Source: CAD feature listing. Evaluate the final solid. Frame: model axes, mm. A direction names the side the tool comes from. Round coordinates to 2 decimals unless told otherwise and drop trailing zeros. Loops run counter-clockwise (first coordinate to the right, second up) from the corner with the lowest first, then second, coordinate; pieces in that order, holes last. Notation, with made-up numbers: (-24, -5.5) - (-1, -5.5) arc R12 ccw to (-1, 12.5) - close; hole circle Ø4 at (3.25, 27.5). An arc over 180 degrees is marked (long way). One line per question, with ' | ' between items. Start each with the question number.
1. Pin query (flat end, axial travel): pin 1 (4 mm diameter, centred on x = 20.5, z = 22, fed in from -Y); pin 2 (1 mm diameter, centred on x = 5, y = 5.5, fed in from +Z); pin 3 (4.5 mm diameter, centred on x = 16.5, y = -2, fed in from +Z); pin 4 (4.5 mm diameter, centred on x = 16.5, y = 0, fed in from -Z). Return the tip coordinate at first contact, or that it passes through.
2. Cut plane B-B (z = 8). Return loops of the section in (x, y).
3. Cut plane A-A (x = 23.5). Return loops of the section in (y, z), then the cut area to 3 significant figures.
4. Mould query, pull axis Y, two halves, no side actions, for faces 1 (the flat face through (15, -2, 27)), 2 (the cylindrical face through (21.32, -7.58, 7.94)), 3 (the flat face through (7, -5.044, 2)), 4 (the flat face through (22.5, -8, 2)). Classes: pulls with the +Y half, pulls with the -Y half, needs draft (parallel to the pull), parting line crosses it, or undercut.
5. Cut plane C-C (y = 5.25). Return loops of the section in (x, z), then the cut area to 3 significant figures.
6. Access query for faces 5 (the flat face through (12, 3, 15)), 6 (the flat face through (15, -12, 1)), 7 (the flat face through (7.5, 1, 2)). Directions: +Z, -Z, +X, -X, +Y, -Y. A direction counts if a zero-diameter tool reaches every point of the face in a straight line with its end or side. Return the directions, or none.
7. Cut plane D-D (x = 27). Return loops of the section in (y, z), then the cut area to 3 significant figures.
8. Ray query, line 1 (Z direction, x = 27.25, y = 3.25); line 2 (Y direction, x = 14.5, z = 7.25); line 3 (Y direction, x = 14.75, z = 1.5). Return the intervals inside material, ascending.
```python
from build123d import *

# Parameters (mm, degrees)
EXTRUDE_1_DEPTH = 1
EXTRUDE_2_DEPTH = 3
SKETCH_3_W      = 15
SKETCH_3_H      = 15
EXTRUDE_3_DEPTH = 3
SKETCH_4_R      = 7.5
EXTRUDE_4_DEPTH = 8
SKETCH_5_R      = 6.6
EXTRUDE_5_DEPTH = 3


with BuildPart() as part:
    # 草图1 → 凸台-拉伸1 (new body)
    with BuildSketch(Plane.XY):
        with BuildLine():
            Line((4.2, 8.956043956), (25.8, 8.956043956))
            ThreePointArc((25.8, 8.956043956), (27, 7.756043956), (28.2, 8.956043956))
            Line((28.2, 8.956043956), (30, 8.956043956))
            Line((30, 8.956043956), (30, -16.043956044))
            Line((30, -16.043956044), (28.2, -16.043956044))
            ThreePointArc((28.2, -16.043956044), (27, -14.843956044), (25.8, -16.043956044))
            Line((25.8, -16.043956044), (4.2, -16.043956044))
            ThreePointArc((4.2, -16.043956044), (3, -14.843956044), (1.8, -16.043956044))
            Line((1.8, -16.043956044), (0, -16.043956044))
            Line((0, -16.043956044), (0, 8.956043956))
            Line((0, 8.956043956), (1.8, 8.956043956))
            ThreePointArc((1.8, 8.956043956), (3, 7.756043956), (4.2, 8.956043956))
        make_face()
    extrude(amount=EXTRUDE_1_DEPTH)

    # 草图2 → 凸台-拉伸2 (add)
    with BuildSketch(Plane.XY.offset(1)):
        with BuildLine():
            Line((6, -2.043956044), (24, -2.043956044))
            ThreePointArc((24, -2.043956044), (25.5, -3.543956044), (24, -5.043956044))
            Line((24, -5.043956044), (6, -5.043956044))
            ThreePointArc((6, -5.043956044), (4.5, -3.543956044), (6, -2.043956044))
        make_face()
    extrude(amount=EXTRUDE_2_DEPTH)

    # 草图3 → 凸台-拉伸3 (add)
    with BuildSketch(Plane.XY.offset(1)):
        with Locations((15, -3.543956044)):
            Rectangle(SKETCH_3_W, SKETCH_3_H)
    extrude(amount=EXTRUDE_3_DEPTH)

    # 草图4 → 凸台-拉伸4 (add)
    with BuildSketch(Plane.XY.offset(4)):
        with Locations(Location((15, -3.543956044, 0), (0, 0, 270))):
            Circle(SKETCH_4_R)
    extrude(amount=EXTRUDE_4_DEPTH)

    # 草图5 → 凸台-拉伸5 (add)
    with BuildSketch(Plane.XY.offset(12)):
        with Locations((15, -3.543956044)):
            Circle(SKETCH_5_R)
    extrude(amount=EXTRUDE_5_DEPTH)

    # 草图7 → 旋转2 (revolve)
    with BuildSketch(Plane(origin=(0, -3.543956044, 0), x_dir=(-1, 0, 0), z_dir=(0, -1, 0)), mode=Mode.PRIVATE) as revolve_2_sk:
        with BuildLine():
            Line((-15, -15), (-7.5, -15))
            Line((-7.5, -15), (-7.5, -27))
            Line((-7.5, -27), (-7.5095257, -28.070803971))
            Line((-7.5095257, -28.070803971), (-7.681219097, -28.070803971))
            ThreePointArc((-7.681219097, -28.070803971), (-8.373062515, -27.290151024), (-9.375, -27))
            Line((-9.375, -27), (-14.500000001, -27))
            ThreePointArc((-14.500000001, -27), (-14.646437925, -27.353569269), (-15, -27.500024563))
            Line((-15, -27.500024563), (-15, -27.000024563))
            Line((-15, -27.000024563), (-15, -22))
            Line((-15, -22), (-15, -15))
        make_face()
    revolve(revolve_2_sk.sketch.rotate(Axis((15, -3.543956044, 22), (0, 0, -1)), 180), axis=Axis((15, -3.543956044, 22), (0, 0, -1)))


solid = part.part
```
Answers follow:
1) pin 1: stops at y = -10.18 | pin 2: stops at z = 1 | pin 3: stops at z = 27.5 | pin 4: stops at z = 0
2) outline: circle Ø15 at (15, -3.54)
3) outline: (-16.04, 0) - (8.96, 0) - (8.96, 1) - (-2.04, 1) - (-2.04, 4) - (-5.04, 4) - (-5.04, 1) - (-16.04, 1) - close | area: 34.0 mm2
4) face 1: undercut | face 2: parting line crosses it | face 3: pulls with the -Y half | face 4: needs draft
5) outline: (0, 0) - (30, 0) - (30, 1) - (0, 1) - close | area: 30.0 mm2
6) face 5: none | face 6: +Z | face 7: +Z, -X, +Y
7) outline: (-14.84, 0) - (7.76, 0) - (7.76, 1) - (-14.84, 1) - close | area: 22.6 mm2
8) line 1: z = 0 to 1 | line 2: y = -11.03 to 3.94 | line 3: y = -11.04 to 3.96
